Check sheet for the modelled part. Datum: model origin and axes. Units: mm. Face numbers are marked on the shaded views. A direction names the side the tool comes from. Round coordinates to 2 decimals unless told otherwise and drop trailing zeros. Write each loop counter-clockwise with the first axis right and the second up, starting at its lowest first coordinate (ties: lowest second). Pieces come first, ordered by that corner, then holes. Notation, with made-up numbers: (50.5, 40) -> (84.5, 40) arc R35 ccw to (84.5, 74) -> close; hole circle Ø7 at (-28, 31). An arc over 180 degrees is marked (long way). Put each result on its own line as item: value. Start each with the question number.
from build123d import *

# Parameters (mm, degrees)
BOSS_EXTRUDE2_DEPTH = 25.4
SKETCH13_R          = 2.54
CUT_EXTRUDE4_DEPTH  = 6.35
SKETCH12_R          = 2.54
CUT_EXTRUDE5_DEPTH  = 6.35
SKETCH14_R          = 2.54
CUT_EXTRUDE6_DEPTH  = 6.35
BOSS_EXTRUDE3_DEPTH = 2.54
FILLET1_R           = 2.54
FILLET2_R           = 2.54
SKETCH18_R          = 3.175
CUT_EXTRUDE7_DEPTH  = 2.54


with BuildPart() as part:
    # Sketch6 → Boss-Extrude2 (new body)
    with BuildSketch(Plane(origin=(0, 0, 0), x_dir=(0, 0, -1), z_dir=(1, 0, 0))):
        Polygon((-13.082661166, -7.52885515), (-5.10893156, -18.225236378), (-17.80893156, -18.225236378), (-17.80893156, -21.061645655), (17.80893156, -21.061645655), (17.80893156, -18.225236378), (5.10893156, -18.225236378), (13.082661166, -7.52885515), align=None)
        with BuildLine():
            Line((7.950045252, -9.731855656), (3.216371131, -16.081855656))
            ThreePointArc((3.216371131, -16.081855656), (0, -19.298226787), (-3.216371131, -16.081855656))
            Line((-3.216371131, -16.081855656), (-7.950045252, -9.731855656))
            Line((-7.950045252, -9.731855656), (-3.81, -9.731855656))
            Line((-3.81, -9.731855656), (3.81, -9.731855656))
            Line((3.81, -9.731855656), (7.950045252, -9.731855656))
        make_face(mode=Mode.SUBTRACT)
    extrude(amount=BOSS_EXTRUDE2_DEPTH)

    # Sketch13 → Cut-Extrude4 (cut)
    with BuildSketch(Plane(origin=(0, -18.225236378, 0), x_dir=(1, 0, 0), z_dir=(0, 1, 0))):
        with Locations(Location((19.05, -13.99893156, 0), (0, 0, 270))):
            Circle(SKETCH13_R)
    extrude(amount=-CUT_EXTRUDE4_DEPTH, mode=Mode.SUBTRACT)

    # Sketch12 → Cut-Extrude5 (cut)
    with BuildSketch(Plane(origin=(0, -18.225236378, 0), x_dir=(1, 0, 0), z_dir=(0, 1, 0))):
        with Locations(Location((6.35, -13.99893156, 0), (0, 0, 270))):
            Circle(SKETCH12_R)
    extrude(amount=-CUT_EXTRUDE5_DEPTH, mode=Mode.SUBTRACT)

    # Sketch14 → Cut-Extrude6 (cut)
    with BuildSketch(Plane(origin=(0, -18.225236378, 0), x_dir=(1, 0, 0), z_dir=(0, 1, 0))):
        with Locations(Location((19.05, 13.99893156, 0), (0, 0, 270))):
            Circle(SKETCH14_R)
        with Locations(Location((6.35, 13.99893156, 0), (0, 0, 270))):
            Circle(SKETCH14_R)
    extrude(amount=-CUT_EXTRUDE6_DEPTH, mode=Mode.SUBTRACT)

    # Sketch6_4 → Boss-Extrude3 (add)
    with BuildSketch(Plane(origin=(0, 0, 0), x_dir=(0, 0, -1), z_dir=(1, 0, 0))):
        with BuildLine():
            Line((7.950045252, -9.731855656), (3.216371131, -16.081855656))
            ThreePointArc((3.216371131, -16.081855656), (0, -19.298226787), (-3.216371131, -16.081855656))
            Line((-3.216371131, -16.081855656), (-7.950045252, -9.731855656))
            Line((-7.950045252, -9.731855656), (-3.81, -9.731855656))
            Line((-3.81, -9.731855656), (3.81, -9.731855656))
            Line((3.81, -9.731855656), (7.950045252, -9.731855656))
        make_face()
    extrude(amount=BOSS_EXTRUDE3_DEPTH)

    # Fillet1
    fillet1_edges = [part.edges().sort_by_distance(p)[0] for p in [
        (12.7, -7.52885515, 13.082661166),
    ]]
    fillet(fillet1_edges, radius=FILLET1_R)

    # Fillet2
    fillet2_edges = [part.edges().sort_by_distance(p)[0] for p in [
        (12.7, -7.52885515, -13.082661166),
    ]]
    fillet(fillet2_edges, radius=FILLET2_R)

    # Sketch18 → Cut-Extrude7 (cut)
    with BuildSketch(Plane.ZY):
        with Locations((0, -16.081855656)):
            Circle(SKETCH18_R)
    extrude(amount=-CUT_EXTRUDE7_DEPTH, mode=Mode.SUBTRACT)


solid = part.part
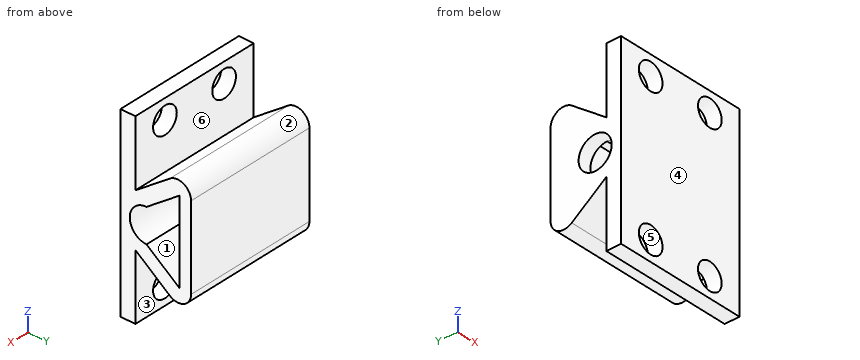
1. Section check A-A, the plane z = 0. Enter the section's corners in (x, y).
2. Section check C-C, the plane y = -20. Enter the section's corners in (x, z), then the cut area to 3 significant figures.
3. Section check B-B, the plane x = 6.35. Enter the section's corners in (y, z), then the cut area to 3 significant figures.
4. Section check D-D, the plane y = -15.25. Enter the section's corners in (x, z).
5. Draft check along Y on the marked faces 4, 5 and 6. Enter one of: released by +Y, released by -Y, zero draft, split by the parting line, or undercut.
6. Gauge pin test, flat ends, axial feed: P1, Ø4, axis at x = 6.35, z = -14, coming from the -Y side; P2, Ø3, axis at x = 7.5, y = -14.5, coming from the +Z side; P3, Ø3, axis at x = 15, z = 9.5, coming from the +Y side; P4, Ø4, axis at x = 15, z = -13.5, coming from the +Y side. Record the tip position at first contact, or that the pin passes through.
7. Access from +Z, -Z, +X, -X, +Y, -Y to the whole of each face (thin tool, end or side, straight path). Record for the marked faces 1, 2 and 3.
8. Material ranges on L1, parallel to Z at x = 17.5, y = -19.5; L2, parallel to Y at x = 4, z = 6.5; L3, parallel to Y at x = 0.7, z = 0, recorded low to high. Write a range as [from, to].
Reply:
1. outline: (0, -21.06) -> (25.4, -21.06) -> (25.4, -19.3) -> (2.54, -19.3) -> (2.54, -19.26) -> (0, -19.26) -> close; (0, -12.91) -> (2.54, -12.91) -> (2.54, -9.73) -> (25.4, -9.73) -> (25.4, -7.53) -> (0, -7.53) -> close
2. outline: (0, -17.81) -> (25.4, -17.81) -> (25.4, 17.81) -> (0, 17.81) -> close; hole circle Ø5.08 at (6.35, -14); hole circle Ø5.08 at (6.35, 14); hole circle Ø5.08 at (19.05, -14); hole circle Ø5.08 at (19.05, 14)
2. area: 824 mm2
3. outline: (-21.06, -17.81) -> (-18.23, -17.81) -> (-18.23, -16.54) -> (-21.06, -16.54) -> close; (-21.06, -11.46) -> (-18.23, -11.46) -> (-18.23, -5.11) -> (-11.59, -10.06) arc R2.54 ccw to (-7.53, -8.02) -> (-7.53, 8.02) arc R2.54 ccw to (-11.59, 10.06) -> (-18.23, 5.11) -> (-18.23, 11.46) -> (-21.06, 11.46) -> close; (-21.06, 16.54) -> (-18.23, 16.54) -> (-18.23, 17.81) -> (-21.06, 17.81) -> close; hole (-16.08, -3.22) -> (-9.73, -7.95) -> (-9.73, 7.95) -> (-16.08, 3.22) arc R3.22 ccw to start
3. area: 168 mm2
4. outline: (0, -7.33) -> (25.4, -7.33) -> (25.4, -3.84) -> (2.54, -3.84) -> (2.54, -3.06) -> (0, -3.06) -> close; (0, 3.06) -> (2.54, 3.06) -> (2.54, 3.84) -> (25.4, 3.84) -> (25.4, 7.33) -> (0, 7.33) -> close
5. face 4: released by -Y
5. face 5: zero draft
5. face 6: undercut
6. P1: passes through
6. P2: stops at z = 9
6. P3: stops at y = -7.53
6. P4: stops at y = -18.23
7. face 1: +X
7. face 2: +Z, +X, -X
7. face 3: -Z, +X, -X
8. L1: z = [-17.81, -16.01], [-11.99, 11.99], [16.01, 17.81]
8. L2: y = [-21.06, -18.23], [-16.36, -11.68], [-9.73, -7.53]
8. L3: y = [-21.06, -19.26], [-12.91, -7.53]
